Autodesk Inventor part; units mm, degrees
ref_plane "YZ Plane" through (0, 0, 0) normal (1, 0, 0) x (0, 1, 0)
ref_plane "XZ Plane" through (0, 0, 0) normal (0, 1, 0) x (-1, 0, 0)
ref_plane "XY Plane" through (0, 0, 0) normal (0, 0, 1) x (1, 0, 0)
sketch "Sketch1" plane through (0, 0, 0) normal (1, 0, 0) x (0, 1, 0)
  line L0 (28.309, -15.6604) -> (71.9614, -15.6604)
  line L1 (28.309, -55.6604) -> (28.309, -15.6604)
  line L2 (28.309, -55.6604) -> (71.9614, -15.6604)
  point P0 (0, 0)
  dimension "d2" = 42.5
  dimension "d3" = 90
  dimension "d4" = 40
extrude "Extrusion1" add sketch "Sketch1" along normal blind 10
sketch "Sketch2" plane through (0, 28.309, -55.6604) normal (0, -1, 0) x (1, 0, 0)
  line L0 (0, 40) -> (0, 0)
  line L1 (0, 0) -> (10, 0)
  line L2 (10, 40) -> (10, 0)
  line L3 (0, 40) -> (10, 40)
  point P0 (0, 55.6604)
extrude "Extrusion2" add sketch "Sketch2" along normal blind 10
sketch "Sketch3" plane through (0, 18.309, -55.6604) normal (0, -1, 0) x (1, 0, 0)
  arc A0 (1, 4) -> (9, 4) centre (5, 4) ccw
  line L0 (9, 4) -> (9, 100)
  arc A1 (9, 100) -> (1, 100) centre (5, 100) ccw
  line L1 (1, 100) -> (1, 4)
  circle A2 centre (5, 100) radius 2
  circle A3 centre (5, 92) radius 2
  circle A4 centre (5, 84) radius 2
  circle A5 centre (5, 76) radius 2
  circle A6 centre (5, 68) radius 2
  circle A7 centre (5, 60) radius 2
  circle A8 centre (5, 52) radius 2
  circle A9 centre (5, 44) radius 2
  circle A10 centre (5, 36) radius 2
  circle A11 centre (5, 28) radius 2
  circle A12 centre (5, 20) radius 2
  circle A13 centre (5, 12) radius 2
  circle A14 centre (5, 4) radius 2
  point P0 (0, 55.6604)
extrude "Extrusion3" cut sketch "Sketch3" against normal blind 10 contours A10 | A14
sketch "Sketch4" plane through (10, 71.9614, -15.6604) normal (0, 0.6755902, -0.7372773) x (-1, 0, 0)
  line L0 (10, -59.2075) -> (10, 0)
  line L1 (10, 0) -> (0, 0)
  line L2 (0, -59.2075) -> (0, 0)
  line L3 (10, -59.2075) -> (0, -59.2075)
  circle A0 centre (5, -10) radius 2
  circle A1 centre (5, -49.2075) radius 2
  point P0 (10, -42.4755)
  dimension "d11" = 4
  dimension "d12" = 4
  dimension "d13" = 10
  dimension "d14" = 10
extrude "Extrusion4" cut sketch "Sketch4" against normal blind 10 contours A0 | A1
sketch "Sketch5" plane through (10, 0, 0) normal (1, 0, 0) x (0, 0, -1)
  line L0 (53.6604, 18.309) -> (53.6604, 28.309)
  line L1 (49.6604, 18.309) -> (49.6604, 28.309)
  line L2 (21.6604, 18.309) -> (21.6604, 28.309)
  line L3 (17.6604, 18.309) -> (17.6604, 28.309)
  line L4 (16.1104, 27.309) -> (23.2104, 27.309)
  line L5 (23.2104, 27.309) -> (23.2104, 22.309)
  line L6 (23.2104, 22.309) -> (16.1104, 22.309)
  line L7 (16.1104, 22.309) -> (16.1104, 27.309)
  line L8 (55.6604, 18.309) -> (15.6604, 18.309)
  line L9 (48.1104, 27.309) -> (55.2104, 27.309)
  line L10 (55.2104, 27.309) -> (55.2104, 22.309)
  line L11 (55.2104, 22.309) -> (48.1104, 22.309)
  line L12 (48.1104, 22.309) -> (48.1104, 27.309)
  line L13 (23.7675, 63.114) -> (16.3947, 56.3581)
  line L14 (21.0651, 66.0632) -> (15.6604, 61.1106)
  line L15 (50.2557, 34.2073) -> (42.8829, 27.4514)
  line L16 (47.5533, 37.1564) -> (40.1805, 30.4005)
  line L17 (17.0688, 64.5036) -> (21.8655, 59.2689)
  line L18 (21.8655, 59.2689) -> (18.1791, 55.891)
  line L19 (18.1791, 55.891) -> (13.3824, 61.1256)
  line L20 (13.3824, 61.1256) -> (17.0688, 64.5036)
  line L21 (55.6604, 28.309) -> (15.6604, 71.9614)
  line L22 (15.6604, 71.9614) -> (15.6604, 18.309)
  line L23 (43.557, 35.5968) -> (48.3537, 30.3621)
  line L24 (48.3537, 30.3621) -> (44.6673, 26.9842)
  line L25 (44.6673, 26.9842) -> (39.8706, 32.2188)
  line L26 (39.8706, 32.2188) -> (43.557, 35.5968)
  point P0 (0, 0)
  dimension "d17" = 7.1
  dimension "d18" = 5
  dimension "d19" = 4
  dimension "d20" = 1.55
  dimension "d21" = 4
  dimension "d22" = 7.1
  dimension "d23" = 5
  dimension "d24" = 4
  dimension "d25" = 1.55
  dimension "d28" = 7.1
  dimension "d29" = 5
  dimension "d30" = 1.55
  dimension "d31" = 4
  dimension "d33" = 7.1
  dimension "d34" = 5
  dimension "d35" = 4
  dimension "d36" = 1.55
sketch "Sketch6" plane through (0, 71.9614, -15.6604) normal (0, 0, 1) x (1, 0, 0)
  ellipse E0 centre (5, -13.5634) end of major axis (5, -16.2761) minor radius 2 (6.7794, -14.8019) -> (3.2206, -14.8019) ccw
  line L0 (6.7794, -14.8019) -> (3.2206, -14.8019)
  line L1 (0, 0) -> (0, -53.6523)
  line L2 (10, -53.6523) -> (0, -53.6523)
  line L3 (10, 0) -> (10, -53.6523)
  line L4 (0, 0) -> (10, 0)
  point P0 (0, -71.9614)
extrude "Extrusion6" add sketch "Sketch6" along normal blind 4 contours L0 E0 | L4 L3 L2 L1
sketch "Sketch7" plane through (10, 28.309, -55.6604) normal (0, 0.6755902, -0.7372773) x (-1, 0, 0)
  circle A0 centre (5, 10) radius 2
  circle A1 centre (5, 49.2075) radius 2
  line L0 (10, 0) -> (10, 59.2075)
  line L1 (10, 59.2075) -> (0, 59.2075)
  line L2 (0, 0) -> (0, 59.2075)
  line L3 (10, 0) -> (0, 0)
  point P0 (10, 16.732)
extrude "Extrusion7" cut sketch "Sketch7" against normal blind 10 contours A1
extrude "Extrusion8" cut sketch "Sketch5" against normal blind 10 contours L11 L1 L9 L0 | L0 L9 L10 L11 | L11 L12 L9 L1 | L6 L3 L4 L2 | L2 L4 L5 L6 | L6 L7 L4 L3 | L17 L18 L19 L13 | L13 L19 L22 L14 L17 | L14 L22 L20 L17 | L19 L20 L22 | L23 L24 L25 L15 | L15 L25 L16 L23 | L16 L25 L26 L23
fillet "Fillet1" radius 2 5 edges at (5, 71.9614, -11.6604) (5, 71.9614, -15.6604) (5, 18.309, -11.6604) (5, 18.309, -55.6604) (5, 28.309, -55.6604)
sketch "Sketch8" plane through (10, 28.8825, -55.1349) normal (0, 0.6755902, -0.7372773) x (-1, 0, 0)
  line L0 (10, 0) -> (0, 0)
  line L1 (10, 0) -> (10, 57.5497)
  line L2 (0, 57.5497) -> (10, 57.5497)
  line L3 (0, 0) -> (0, 57.5497)
  circle A0 centre (5, 48.4297) radius 2
  circle A1 centre (5, 9.2222) radius 2
  line L4 (0, 60.3064) -> (10, 60.3064)
  line L5 (10, -7.3248) -> (0, -7.3248)
  line L6 (0, 60.3064) -> (10, 60.3064)
  line L7 (10, 60.3064) -> (10, -7.3248)
  line L8 (10, -7.3248) -> (0, -7.3248)
  line L9 (0, -7.3248) -> (0, 60.3064)
  line L10 (0, -1.3512) -> (10, -1.3512)
  point P0 (10, 15.9542)
  dimension "d44" = 10
  dimension "d45" = 4
  dimension "d46" = 9.8766
  dimension "d47" = 61.6575
  dimension "d48" = 39.2075
equation "\"d14\" = d13"
equation "\"d20\" = -0.5 * d19 + 0.5 * d17"
equation "\"d24\" = d21"
equation "\"d25\" = d20"
equation "\"d28\" = d17"
equation "\"d29\" = d18"
equation "\"d30\" = d20"
equation "\"d31\" = d21"
equation "\"d35\" = d21"
equation "\"d36\" = d20"
properties part number "intake plate holder"
The listing builds one solid part. Answer for the finished solid, in the listing's coordinates (mm). A direction names the side the tool comes from. Round coordinates to 2 decimals unless told otherwise and drop trailing zeros. Order: outer loops, then holes, each group sorted by start corner. A loop starts at its lowest first (then second) coordinate and runs counter-clockwise, first axis right, second up. Notation, with made-up numbers: (70.25, 59) - (86.25, 59) arc R17 cw to (86.25, 74) - close; hole circle Ø5 at (21.25, 21.5). An arc over 180 degrees is marked (long way). Put each result on its own line as item: value. Start each with the question number.
(1) Determine the mould class of faces 1 (the cylindrical face through (3.153, 62.692, -21.48)), 2 (the cylindrical face through (4.74, 27.802, -49.677)), 3 (the flat face through (7.29, 33.02, -45.92)), 4 (the cylindrical face through (4.93, 18.88, -12.26)) for opening direction Y: released by +Y, released by -Y, zero draft, split by the parting line, or undercut.
(2) For faces 5 (the cylindrical face through (4.74, 20.281, -17.677)), 6 (the flat face through (5, 24, -55.66)), 7 (the flat face through (7.292, 29.565, -42.303)), determine the directions among +Z, -Z, +X, -X, +Y, -Y from which every point of the face is accessible in a straight line to the end or side of a thin tool.
(3) Straight lines are drawn through the part: probe 1 along Z at (x, y) = (5, 20.2); probe 2 along Z at (x, y) = (5, 27.95); probe 3 along Z at (x, y) = (5, 19.7). For each, find the intervals that lie inside material, in ascending order. Write a range as from..to.
(4) Given P1, Ø3.5, axis at x = 3, z = -21, coming from the +Y side; P2, Ø4, axis at x = 1.5, z = -32, coming from the +Y side; P3, Ø3.5, axis at x = 5, z = -19.66, coming from the +Y side, each flat-ended and moving along its own axis, determine where each tip first touches the part or whether it passes through.
(5) Find section A-A (y = 55). Give the vertices of the cut face in (x, z).
Reply:
1. face 1: undercut
1. face 2: zero draft
1. face 3: undercut
1. face 4: released by -Y
2. face 5: -Y
2. face 6: -Z, +X, -X, +Y, -Y
2. face 7: +X, -X
3. probe 1: -55.66..-53.66, -49.66..-21.66, -17.66..-11.66
3. probe 2: -55.62..-53.66, -49.66..-45.72, -43.78..-43.43, -42.42..-21.66, -17.66..-11.66
3. probe 3: -55.57..-53.66, -49.66..-21.66, -17.66..-11.76
4. P1: y = 68.04
4. P2: y = 56.31
4. P3: y = 69.51
5. outline: (0, -31.2) - (10, -31.2) - (10, -11.66) - (0, -11.66) - close
